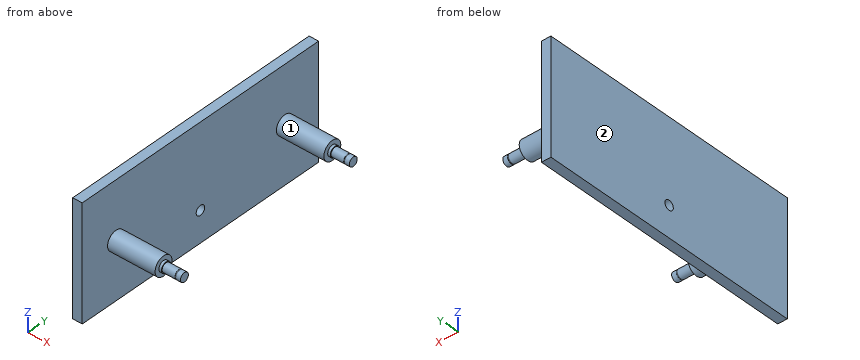
from build123d import *

# Parameters (mm, degrees)
F0_W      = 355.6
F0_H      = 152.4
F1_DEPTH  = 12.7
F3_DEPTH  = 63.5
F4_R      = 6.9999987
F5_DEPTH  = 3.50012
F6_R      = 6.9999987
F7_DEPTH  = 3.50012
F8_R      = 6.0000007
F9_DEPTH  = 16.9999914
F10_R     = 6.0000007
F11_DEPTH = 16.9999914
F12_R     = 5.74999993
F13_DEPTH = 1.10000034
F14_R     = 5.74999993
F15_DEPTH = 1.10000034
F16_R     = 6.0000007
F17_DEPTH = 6.35
F18_R     = 6.0000007
F19_DEPTH = 6.35
F20_R     = 6.35
F21_DEPTH = 25.4


with BuildPart() as f1:
    # F0 (on Right) → F1 (new body)
    with BuildSketch(Plane.YZ):
        with Locations((177.8, 76.2)):
            Rectangle(F0_W, F0_H)
    extrude(amount=F1_DEPTH)

    # F2 (on face) → F3 (join)
    with BuildSketch(Plane.YZ.offset(12.7)):
        with BuildLine():
            ThreePointArc((63.5, 76.2), (50.8, 88.9), (38.1, 76.2))
            Line((38.1, 76.2), (63.5, 76.2))
        make_face()
        with BuildLine():
            ThreePointArc((317.5, 76.2), (304.8, 88.9), (292.1, 76.2))
            Line((292.1, 76.2), (317.5, 76.2))
        make_face()
        with BuildLine():
            Line((317.5, 76.2), (292.1, 76.2))
            ThreePointArc((292.1, 76.2), (304.8, 63.5), (317.5, 76.2))
        make_face()
        with BuildLine():
            Line((63.5, 76.2), (38.1, 76.2))
            ThreePointArc((38.1, 76.2), (50.8, 63.5), (63.5, 76.2))
        make_face()
    extrude(amount=F3_DEPTH)

    # F4 (on face) → F5 (join)
    with BuildSketch(Plane.YZ.offset(76.2)):
        with Locations((50.8, 76.2)):
            Circle(F4_R)
    extrude(amount=F5_DEPTH)

    # F6 (on face) → F7 (join)
    with BuildSketch(Plane.YZ.offset(76.2)):
        with Locations((304.8, 76.2)):
            Circle(F6_R)
    extrude(amount=F7_DEPTH)

    # F8 (on face) → F9 (join)
    with BuildSketch(Plane.YZ.offset(79.70012)):
        with Locations((50.8, 76.2)):
            Circle(F8_R)
    extrude(amount=F9_DEPTH)

    # F10 (on face) → F11 (join)
    with BuildSketch(Plane.YZ.offset(79.70012)):
        with Locations((304.8, 76.2)):
            Circle(F10_R)
    extrude(amount=F11_DEPTH)

    # F12 (on face) → F13 (join)
    with BuildSketch(Plane.YZ.offset(96.7001114)):
        with Locations((50.8, 76.2)):
            Circle(F12_R)
    extrude(amount=F13_DEPTH)

    # F14 (on face) → F15 (join)
    with BuildSketch(Plane.YZ.offset(96.7001114)):
        with Locations((304.8, 76.2)):
            Circle(F14_R)
    extrude(amount=F15_DEPTH)

    # F16 (on face) → F17 (join)
    with BuildSketch(Plane.YZ.offset(97.80011174)):
        with Locations((50.8, 76.2)):
            Circle(F16_R)
    extrude(amount=F17_DEPTH)

    # F18 (on face) → F19 (join)
    with BuildSketch(Plane.YZ.offset(97.80011174)):
        with Locations((304.8, 76.2)):
            Circle(F18_R)
    extrude(amount=F19_DEPTH)

    # F20 (on face) → F21 (cut)
    with BuildSketch(Plane.YZ.offset(12.7)):
        with Locations((177.8, 41.275)):
            Circle(F20_R)
    extrude(amount=-F21_DEPTH, mode=Mode.SUBTRACT)


solid = f1.part
Model file for the job. Use its own axes, mm. Face numbers are marked on the shaded views. Give positions to 0.01 mm unless a question says otherwise; leave off trailing zeros. Order: outer loops, then holes, each group sorted by start corner. A loop starts at its lowest first (then second) coordinate and runs counter-clockwise, first axis right, second up. Notation, with made-up numbers: M 44,12.25 L 85,12.25 A29 ccw 85,49.25 Z; hole C 51.25,44 d4. An arc over 180 degrees is marked long. Write item = value, one per line.
Q1. Flat gauge pin, fed straight in: pin 1 (1 mm diameter, centred on y = 187.5, z = 78.5, fed in from +X). Where does the tip first touch, or does it go through?
Derived:
pin_1 = 12.7
Q2. Cut at B-B, the plane y = 50.8. List the corners of the cut face in (x, z), then the cut area to 3 significant figures.
Derived:
outline = M 0,0 L 12.7,0 L 12.7,63.5 L 76.2,63.5 L 76.2,69.2 L 79.7,69.2 L 79.7,70.2 L 96.7,70.2 L 96.7,70.45 L 97.8,70.45 L 97.8,70.2 L 104.15,70.2 L 104.15,82.2 L 97.8,82.2 L 97.8,81.95 L 96.7,81.95 L 96.7,82.2 L 79.7,82.2 L 79.7,83.2 L 76.2,83.2 L 76.2,88.9 L 12.7,88.9 L 12.7,152.4 L 0,152.4 Z
area = 3,890 mm2
Q3. Cut at C-C, the plane x = 26.5. List the corners of the cut face in (y, z).
Derived:
outline = C 50.8,76.2 d25.4; C 304.8,76.2 d25.4
Q4. Two-plate mould, pull along Y, no slides. Class the marked faces 1 and 2: pulls with the +Y half, pulls with the -Y half, needs draft (parallel to the pull), parting line crosses it, or undercut.
Derived:
face_1 = undercut
face_2 = needs draft
Q5. Cut at A-A, the plane y = 177.8. List the corners of the cut face in (x, z) (3 decimals).
Derived:
outline = M 0,0 L 12.7,0 L 12.7,34.925 L 0,34.925 Z; M 0,47.625 L 12.7,47.625 L 12.7,152.4 L 0,152.4 Z
Q6. Cut at D-D, the plane z = 101. List the corners of the cut face in (x, y).
Derived:
outline = M 0,0 L 12.7,0 L 12.7,355.6 L 0,355.6 Z
Q7. Drill centre lines: line 1 (Z direction, x = 10, y = 177); line 2 (Z direction, x = 4, y = 177.8) (3 decimals); line 3 (X direction, y = 164.5, z = 27). Where is each one in solid material? Low to high. Write a range as [from, to].
Derived:
line_1 = [0, 34.98], [47.57, 152.4]
line_2 = [0, 34.925], [47.625, 152.4]
line_3 = [0, 12.7]
